Geometry: final body of the model. Coordinates: model frame, mm. Give positions to 0.01 mm unless a question says otherwise; leave off trailing zeros. Order: outer loops, then holes, each group sorted by start corner. A loop starts at its lowest first (then second) coordinate and runs counter-clockwise, first axis right, second up. Notation, with made-up numbers: (64, -28.5) -> (108, -28.5) arc R21 ccw to (108, -15.5) -> close; hole circle Ø1 at (27, -14). An arc over 180 degrees is marked (long way). One line per item, written item: value. Start each with the question number.
Autodesk Inventor part; units mm, degrees
ref_plane "YZ Plane" through (0, 0, 0) normal (1, 0, 0) x (0, 1, 0)
ref_plane "XZ Plane" through (0, 0, 0) normal (0, 1, 0) x (-1, 0, 0)
ref_plane "XY Plane" through (0, 0, 0) normal (0, 0, 1) x (1, 0, 0)
sketch "Sketch1" plane through (0, 0, 0) normal (0, 1, 0) x (-1, 0, 0)
  line L0 (0, 0) -> (0, 15)
  line L1 (0, 15) -> (-30, 15)
  line L2 (-30, 15) -> (-30, 0)
  line L3 (-30, 0) -> (0, 0)
  line L4 (0, 0) -> (-21.2132, -21.2132)
  line L5 (0, 0) -> (30, 0) construction
  line L6 (-21.2132, -21.2132) -> (-31.8198, -10.6066)
  line L7 (-31.8198, -10.6066) -> (-21.2132, 0)
  line L8 (0, 15) -> (-21.2132, 36.2132)
  line L9 (0, 15) -> (30, 15) construction
  line L10 (-21.2132, 36.2132) -> (-31.8198, 25.6066)
  line L11 (-31.8198, 25.6066) -> (-21.2132, 15)
  dimension "d0" = 15
  dimension "d1" = 30
  dimension "d2" = 30
  dimension "d3" = 135
  dimension "d4" = 15
  dimension "d5" = 30
  dimension "d6" = 135
extrude "Extrusion1" add sketch "Sketch1" along normal blind 3
sketch "Sketch2" plane through (0, 3, 0) normal (0, 1, 0) x (1, 0, 0)
  circle A0 centre (21.2132, -25.6066) radius 1.75
  circle A1 centre (15.9099, -20.3033) radius 1.75
  circle A2 centre (15, -7.5) radius 1.75
  circle A3 centre (21.2132, 10.6066) radius 1.75
  circle A4 centre (15.9099, 5.3033) radius 1.75
  circle A5 centre (7.5, -7.5) radius 1.75
  circle A6 centre (22.5, -7.5) radius 1.75
  line L0 (31.8198, -25.6066) -> (21.2132, -15)
  line L1 (30, 0) -> (21.2132, 0)
  line L2 (21.2132, 0) -> (31.8198, 10.6066)
  line L3 (21.2132, -36.2132) -> (31.8198, -25.6066)
  line L4 (30, -15) -> (30, 0)
  line L5 (0, 0) -> (0, -15)
  line L6 (31.8198, 10.6066) -> (21.2132, 21.2132)
  dimension "d9" = 3.5
  dimension "d10" = 3.5
  dimension "d11" = 3.5
  dimension "d12" = 3.5
  dimension "d13" = 3.5
  dimension "d14" = 3.5
  dimension "d15" = 3.5
  dimension "d16" = 7.5
  dimension "d18" = 7.5
  dimension "d19" = 7.5
  dimension "d20" = 7.5
  dimension "d21" = 7.5
  dimension "d22" = 7.5
  dimension "d23" = 7.5
  dimension "d24" = 7.5
  dimension "d26" = 15
  dimension "d27" = 7.5
  dimension "d28" = 15
  dimension "d29" = 7.5
  dimension "d30" = 15
  dimension "d31" = 7.5
extrude "Extrusion2" cut sketch "Sketch2" against normal through all
fillet "Fillet1" radius 2 10 edges at (21.2132, 1.5, -21.2132) (31.8198, 1.5, -10.6066) (21.2132, 1.5, 0) (30, 1.5, 0) (30, 1.5, 15) (21.2132, 1.5, 15) (31.8198, 1.5, 25.6066) (21.2132, 1.5, 36.2132) (0, 1.5, 15) (0, 1.5, 0)
equation "\"d16\" = a"
equation "\"d18\" = a"
equation "\"d19\" = a"
equation "\"d20\" = a"
equation "\"d21\" = a"
equation "\"d22\" = a"
equation "\"d23\" = a"
equation "\"d24\" = a"
equation "\"d27\" = a"
equation "\"d29\" = a"
equation "\"d31\" = a"
equation "\"a\" = 7.5"
properties part number "45 degree angle bracket"
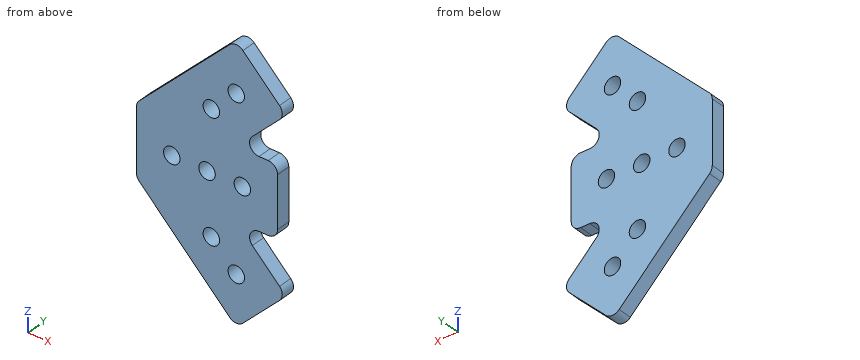
1. Pin query (flat end, axial travel): P1, Ø2, axis at x = 27.5, z = 11.5, coming from the -Y side; P2, Ø3, axis at x = 21.21, z = 25.61, coming from the +Y side; P3, Ø1.6, axis at x = 27, y = 1.5, coming from the +Z side; P4, Ø1, axis at x = 26.5, y = 1.5, coming from the -Z side. Return the tip coordinate at first contact, or that it passes through.
2. Cut plane D-D, the plane y = 1.7. Return loops of the section in (x, z).
3. Material intervals for L1, parallel to X at y = 2.4, z = 7.5; L2, parallel to Z at x = 15, y = 1.05; L3, parallel to Z at x = 28, y = 1.75, sorted ascending. Write a range as [from, to].
4. Cut plane B-B, the plane x = 7.5. Return loops of the section in (y, z), then the cut area to 3 significant figures.
5. Cut plane C-C, the plane x = 15. Return loops of the section in (y, z).
6. Cut plane A-A, the plane z = 7.5. Return loops of the section in (x, y), then the cut area to 3 significant figures.
Answers follow:
1. P1: stops at y = 0
1. P2: passes through
1. P3: stops at z = 31.23
1. P4: stops at z = -16.43
2. outline: (0, 0.83) arc R2 ccw to (0.59, -0.59) -> (19.8, -19.8) arc R2 ccw to (22.63, -19.8) -> (30.41, -12.02) arc R2 ccw to (30.41, -9.19) -> (24.63, -3.41) arc R2 cw to (26.04, 0) -> (28, 0) arc R2 ccw to (30, 2) -> (30, 13) arc R2 ccw to (28, 15) -> (26.04, 15) arc R2 cw to (24.63, 18.41) -> (30.41, 24.19) arc R2 ccw to (30.41, 27.02) -> (22.63, 34.8) arc R2 ccw to (19.8, 34.8) -> (0.59, 15.59) arc R2 ccw to (0, 14.17) -> close; hole circle Ø3.5 at (7.5, 7.5); hole circle Ø3.5 at (15, 7.5); hole circle Ø3.5 at (15.91, -5.3); hole circle Ø3.5 at (15.91, 20.3); hole circle Ø3.5 at (21.21, -10.61); hole circle Ø3.5 at (21.21, 25.61); hole circle Ø3.5 at (22.5, 7.5)
3. L1: x = [0, 5.75], [9.25, 13.25], [16.75, 20.75], [24.25, 30]
3. L2: z = [-15, -6.8], [-3.81, 5.75], [9.25, 18.81], [21.8, 30]
3. L3: z = [-14.43, -6.79], [0, 15], [21.79, 29.43]
4. outline: (0, -7.5) -> (3, -7.5) -> (3, 5.75) -> (0, 5.75) -> close; (0, 9.25) -> (3, 9.25) -> (3, 22.5) -> (0, 22.5) -> close
4. area: 79.5 mm²
5. outline: (0, -15) -> (3, -15) -> (3, -6.8) -> (0, -6.8) -> close; (0, -3.81) -> (3, -3.81) -> (3, 5.75) -> (0, 5.75) -> close; (0, 9.25) -> (3, 9.25) -> (3, 18.81) -> (0, 18.81) -> close; (0, 21.8) -> (3, 21.8) -> (3, 30) -> (0, 30) -> close
6. outline: (0, 0) -> (5.75, 0) -> (5.75, 3) -> (0, 3) -> close; (9.25, 0) -> (13.25, 0) -> (13.25, 3) -> (9.25, 3) -> close; (16.75, 0) -> (20.75, 0) -> (20.75, 3) -> (16.75, 3) -> close; (24.25, 0) -> (30, 0) -> (30, 3) -> (24.25, 3) -> close
6. area: 58.5 mm²
